Could you check a few things on this model? Use its own coordinates, in mm. Face numbers are marked on the shaded views. Give positions to 0.01 mm unless a question says otherwise; leave off trailing zeros. Loops run counter-clockwise (first coordinate to the right, second up) from the corner with the lowest first, then second, coordinate; pieces in that order, holes last. Notation, with made-up numbers: M 25.5,-26 L 52.5,-26 A26 ccw 52.5,7 Z; hole C 44,-16.75 d4. An arc over 180 degrees is marked long. Use CSV: the item, a comma, the result in double quotes.
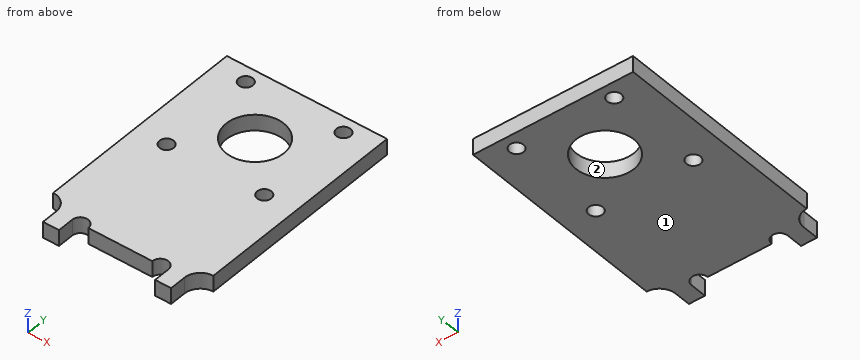
```python
from build123d import *

# Parameters (mm, degrees)
F1_R     = 2.2
F1_R_2   = 9
F2_DEPTH = 5


# Not quite as in the source:
# - a feature names something its author has since deleted; it is built from what else it names


with BuildPart() as f2:
    # F1 (on Top) → F2 (new body)
    with BuildSketch(Plane.XY):
        with BuildLine():
            Line((25, 20), (20, 20))
            Line((20, 20), (-20, 20))
            Line((-20, 20), (-25, 20))
            Line((-25, 20), (-25, -46.9))
            ThreePointArc((-25, -46.9), (-21.4644660941, -48.3644660941), (-20, -51.9))
            Line((-20, -51.9), (-20, -57))
            Line((-20, -57), (-15, -57))
            Line((-15, -57), (-15, -51.9))
            ThreePointArc((-15, -51.9), (-12.5, -49.4), (-10, -51.9))
            Line((-10, -51.9), (0, -51.9))
            Line((0, -51.9), (10, -51.9))
            ThreePointArc((10, -51.9), (12.5, -49.4), (15, -51.9))
            Line((15, -51.9), (15, -57))
            Line((15, -57), (20, -57))
            Line((20, -57), (20, -51.9))
            ThreePointArc((20, -51.9), (21.4644660941, -48.3644660941), (25, -46.9))
            Line((25, -46.9), (25, 20))
        make_face()
        with Locations((-15.25, -15.25)):
            Circle(F1_R, mode=Mode.SUBTRACT)
        with Locations((-15.25, 15.25)):
            Circle(F1_R, mode=Mode.SUBTRACT)
        Circle(F1_R_2, mode=Mode.SUBTRACT)
        with Locations((15.25, -15.25)):
            Circle(F1_R, mode=Mode.SUBTRACT)
        with Locations((15.25, 15.25)):
            Circle(F1_R, mode=Mode.SUBTRACT)
    extrude(amount=F2_DEPTH)


solid = f2.part
```
1. I want a section at A-A, the plane y = 0. List the corners of the cut face in (x, z) for me, then the cut area to 3 significant figures.
Outcome:
outline,"M -25,0 L -9,0 L -9,5 L -25,5 Z; M 9,0 L 25,0 L 25,5 L 9,5 Z"
area,"160 mm2"
2. I want a section at B-B, the plane z = 2.9. List the corners of the cut face in (x, y) for me, then the cut area to 3 significant figures.
Outcome:
outline,"M -25,-46.9 A5 cw -20,-51.9 L -20,-57 L -15,-57 L -15,-51.9 A2.5 cw -10,-51.9 L 10,-51.9 A2.5 cw 15,-51.9 L 15,-57 L 20,-57 L 20,-51.9 A5 cw 25,-46.9 L 25,20 L -25,20 Z; hole C -15.25,-15.25 d4.4; hole C -15.25,15.25 d4.4; hole C 0,0 d18; hole C 15.25,-15.25 d4.4; hole C 15.25,15.25 d4.4"
area,"3,270 mm2"
3. I want a section at C-C, the plane y = -15.25. List the corners of the cut face in (x, z) for me, then the cut area to 3 significant figures.
Outcome:
outline,"M -25,0 L -17.45,0 L -17.45,5 L -25,5 Z; M -13.05,0 L 13.05,0 L 13.05,5 L -13.05,5 Z; M 17.45,0 L 25,0 L 25,5 L 17.45,5 Z"
area,"206 mm2"
4. If we mould it in two halves opening along X, with no side actions, what happens to the marked faces 1 and 2? For each: +X half, -X half, draft (parallel to the pull), parting line (faces both ways), or undercut.
Outcome:
face 1,"draft"
face 2,"undercut"
5. I'm going to push flat-ended pins straight in: pin 1 Ø2.5 at (x, z) = (2.5, 3.5) entering from -Y; pin 2 Ø1 at (x, y) = (-14, -14.5) entering from +Z; pin 3 Ø2.5 at (y, z) = (-53.5, 2.5) entering from +X. Where does each tip first touch, or does it pass through?
Outcome:
pin 1,"y = -51.9"
pin 2,"through"
pin 3,"x = 20"
6. I want a section at D-D, the plane x = -4. List the corners of the cut face in (y, z) for me, then the cut area to 3 significant figures.
Outcome:
outline,"M -51.9,0 L -8.06,0 L -8.06,5 L -51.9,5 Z; M 8.06,0 L 20,0 L 20,5 L 8.06,5 Z"
area,"279 mm2"
7. Please list where these lines run through material, in increasing order: line 1 (Y direction, x = -15.25, z = 3.2); line 2 (Y direction, x = 0.5, z = 1); line 3 (X direction, y = -53, z = 1.45).
Outcome:
line 1,"-57 to -17.45, -13.05 to 13.05, 17.45 to 20"
line 2,"-51.9 to -8.99, 8.99 to 20"
line 3,"-20 to -15, 15 to 20"
